```python
from build123d import *

# Parameters (mm, degrees)
F1_DEPTH = 3
F2_R     = 1.49999


# Not quite as in the source:
# - a fillet or chamfer is up to 0.001 mm smaller than in the source, because OpenCascade refuses the exact size


with BuildPart() as f1:
    # F0 (on Top) → F1 (new body)
    with BuildSketch(Plane.XY):
        Polygon((20, 60), (0, 0), (20, 0), (70, 60), align=None)
    extrude(amount=F1_DEPTH)

    # F2 (radius 1.5 in the source; OpenCascade refuses exactly that, so slightly less here)
    f2_edges = [f1.edges().sort_by_distance(p)[0] for p in [
        (45, 60, 3),
        (10, 30, 0),
        (10, 30, 3),
        (45, 60, 0),
        (20, 60, 1.5),
    ]]
    fillet(f2_edges, radius=F2_R)


solid = f1.part
```
Here's how the part is built. I have some questions about the finished solid (model axes, mm). Give positions to 0.01 mm unless a question says otherwise; leave off trailing zeros. Write each loop counter-clockwise with the first axis right and the second up, starting at its lowest first coordinate (ties: lowest second). Pieces come first, ordered by that corner, then holes.
(1) Will this pin go through, and if not, where does the flat tip stop? pin 1 (8 mm diameter, centred on x = 41.5, y = 17.5, fed in from -Z).
Output values:
pin 1: passes through
(2) Imagine slicing it at B-B, the plane z = 2.4. Write out the boundary of the cut face in (x, y).
Output values:
outline: (0.32, 0) - (20, 0) - (69.75, 59.7) - (21.08, 59.7) arc R1.2 ccw to (19.94, 58.88) - close
(3) If I drill on L1, parallel to Y at x = 24, z = 2.45; L2, parallel to X at y = 35.5, z = 1.8; L3, parallel to X at y = 11.5, z = 1.9, over which ranges is the centre line in solid material (lowest first)?
Output values:
L1: y = 4.8 to 59.66
L2: x = 11.87 to 49.58
L3: x = 3.89 to 29.58
